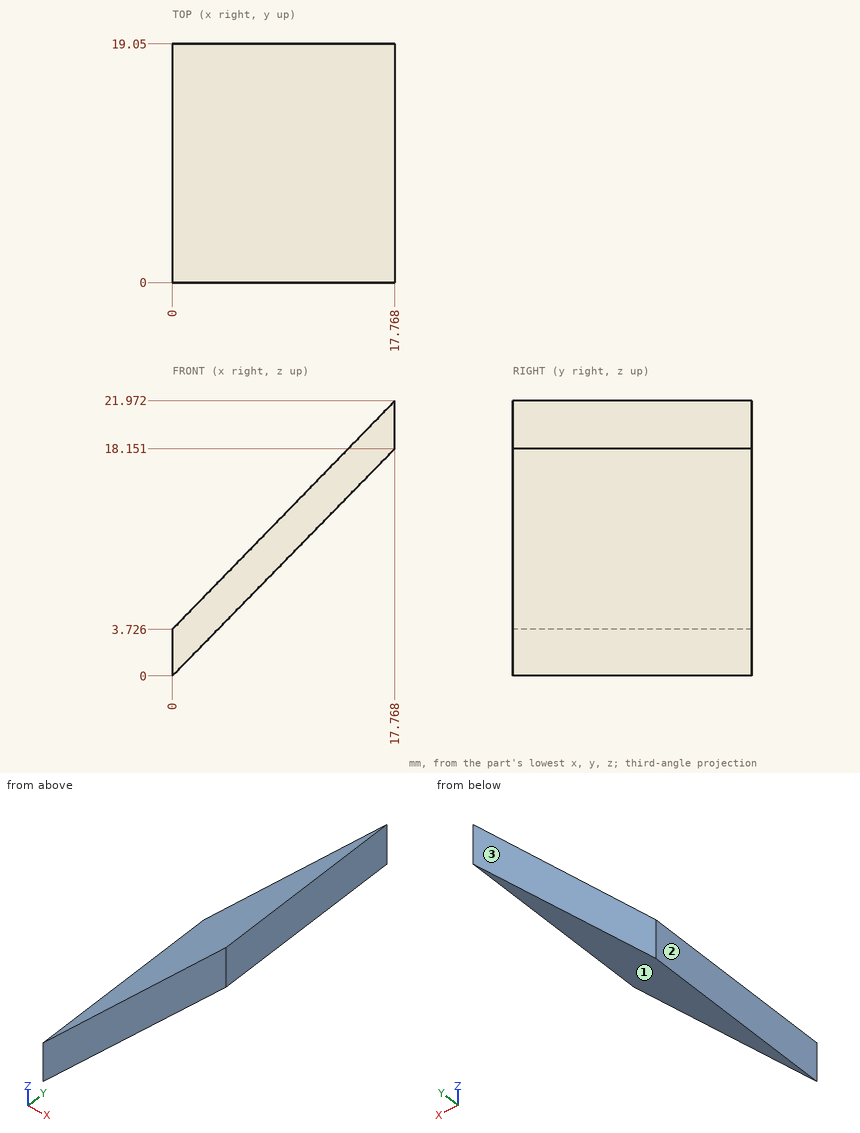
Study the drawing (mm; zero at the part's minimum x, y, z) and answer. Give positions to 0.01 mm unless a question says otherwise; leave off trailing zeros. Write item = value, one per line.
Q1. Consider line 1 along X through (y, z) = (5.25, 10); line 2 along Z through (x, y) = (13.5, 4.5); line 3 along X through (y, z) = (5.5, 9.5) (1 decimal). Determine where each line is inside the solid, lowest interval first.
Computed values:
line_1 = 6.11 to 9.79
line_2 = 13.79 to 17.59
line_3 = 5.6 to 9.3
Q2. Flat-ended cylindrical pins translate along their axes: pin 1 Ø10 at (x, y) = (15, 17) entering from -Z (1 decimal); pin 2 Ø10 at (y, z) = (15.5, 7.5) entering from +X; pin 3 Ø1 at (x, y) = (8, 15.5) entering from +Z (1 decimal). Find the tip coordinate at first contact, or state that the pin passes through.
Computed values:
pin_1 = 10.2
pin_2 = 12.24
pin_3 = 12.5
Q3. For a pull along X with two mould halves and no side action, classify the marked faces 1, 2 and 3 as pulls with the +X half, pulls with the -X half, needs draft (parallel to the pull), parting line crosses it, or undercut.
Computed values:
face_1 = pulls with the +X half
face_2 = pulls with the -X half
face_3 = needs draft
